The listing builds one solid part. Answer for the finished solid, in the listing's coordinates (mm). Face numbers are marked on the shaded views. A direction names the side the tool comes from. Give positions to 0.01 mm unless a question says otherwise; leave off trailing zeros. Write each loop counter-clockwise with the first axis right and the second up, starting at its lowest first coordinate (ties: lowest second). Pieces come first, ordered by that corner, then holes. Notation, with made-up numbers: (-15.5, -17.5) -> (-1.5, -17.5) arc R21 cw to (-1.5, 11.5) -> close; hole circle Ø9 at (34, -2.75). An arc over 180 degrees is marked (long way). Use CSV: the item, a comma, the result in double quotes. Start each with the question number.
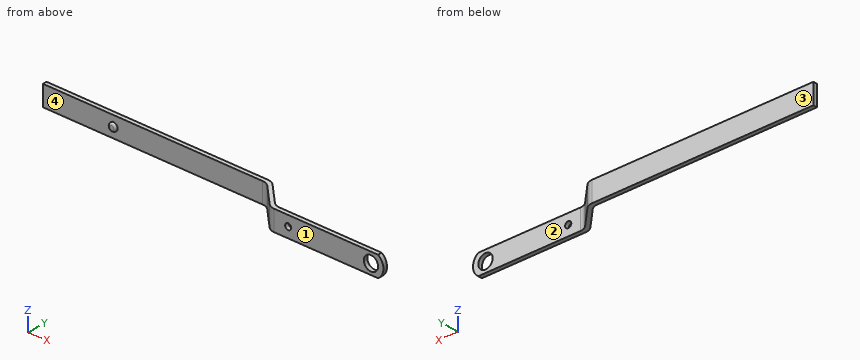
from build123d import *

# Parameters (mm, degrees)
SKETCH3_W           = 20
SKETCH3_H           = 4
FILLET1_R           = 10
BOSS_EXTRUDE1_DEPTH = 4
SKETCH4_4_R         = 7
SKETCH4_4_R_2       = 3
CUT_EXTRUDE6_DEPTH  = 4
SKETCH5_R           = 4
BOSS_EXTRUDE2_DEPTH = 2
FILLET4_R           = 2


with BuildPart() as part:
    # Sweep1: sweep along a path in Sketch2
    with BuildLine(Plane.XY) as sweep1_path:
        Line((105, 0), (0, 0))
        Line((0, 0), (-24.748737342, 24.748737342))
        Line((-24.748737342, 24.748737342), (-159.748737342, 24.748737342))
        Line((-159.748737342, 24.748737342), (-244.748737342, 24.748737342))
    # Sketch3 → Sweep1 (sweep)
    with BuildSketch(Plane(origin=(105, 0, 0), x_dir=(0, 0, -1), z_dir=(1, 0, 0))):
        Rectangle(SKETCH3_W, SKETCH3_H)
    sweep(path=sweep1_path.line, transition=Transition.RIGHT)

    # Fillet1
    fillet1_edges = [part.edges().sort_by_distance(p)[0] for p in [
        (-0.828427125, -2, 0),
        (0.828427125, 2, 0),
        (-23.920310217, 26.748737342, 0),
        (-25.577164466, 22.748737342, 0),
    ]]
    fillet(fillet1_edges, radius=FILLET1_R)

    # Sketch4 → Boss-Extrude1 (add)
    with BuildSketch(Plane(origin=(0, 2, 0), x_dir=(1, 0, 0), z_dir=(0, 1, 0))):
        with BuildLine():
            ThreePointArc((105, -10), (110.206555616, 0), (105, 10))
            Line((105, 10), (105, 0))
            Line((105, 0), (105, -10))
        make_face()
    extrude(amount=-BOSS_EXTRUDE1_DEPTH)

    # Sketch4<4> → Cut-Extrude6 (cut)
    with BuildSketch(Plane(origin=(0, 2, 0), x_dir=(1, 0, 0), z_dir=(0, 1, 0))):
        with Locations(Location((98, 0, 0), (0, 0, 270))):
            Circle(SKETCH4_4_R)
        with Locations(Location((17, 0, 0), (0, 0, 270))):
            Circle(SKETCH4_4_R_2)
    extrude(amount=-CUT_EXTRUDE6_DEPTH, mode=Mode.SUBTRACT)

    # Sketch5 → Boss-Extrude2 (add)
    with BuildSketch(Plane.XZ.offset(-22.748737342)):
        with Locations(Location((-175.748737342, 0, 0), (0, 0, 180))):
            Circle(SKETCH5_R)
    extrude(amount=BOSS_EXTRUDE2_DEPTH)

    # Fillet4
    fillet4_edges = [part.edges().sort_by_distance(p)[0] for p in [
        (-171.748737342, 20.748737342, 0),
    ]]
    fillet(fillet4_edges, radius=FILLET4_R - 0.0001)  # a hair under: the kernel refuses the full size


solid = part.part
Q1. Section A-A on x = 17 is taken. Give the vertices of the cut face in (y, z), then the cut area to 3 significant figures.
Q2. Section B-B on x = 98 is taken. Give the vertices of the cut face in (y, z).
Q3. Straight lines are drawn through the part: L1, parallel to X at y = 0.7, z = 0; L2, parallel to X at y = 0.25, z = 0; L3, parallel to Y at x = -132, z = -8. For each, find the intervals that lie inside material, in ascending order.
Q4. Section C-C on x = -183.5 is taken. Give the vertices of the cut face in (y, z), then the cut area to 3 significant figures.
Q5. Flat-ended cylindrical pins translate along their axes: pin 1 Ø1 at (y, z) = (7.5, -7.5) entering from -X; pin 2 Ø12 at (y, z) = (10, 4) entering from +X; pin 3 Ø3 at (y, z) = (15.5, 1) entering from +X. Find the tip coordinate at first contact, or state that the pin passes through.
Q6. Section D-D on y = 9.75 is taken. Give the vertices of the cut face in (x, z), then the cut area to 3 significant figures.
Q7. The mould has two halves that part along X. Classify the marked faces 3 and 4: +X half, -X half, draft (parallel to the pull), parting line (faces both ways), or undercut.
Q8. For the marked faces 1 and 2, determine the directions among +Z, -Z, +X, -X, +Y, -Y from which every point of the face is accessible in a straight line to the end or side of a thin tool.
Output:
1,outline,"(-2, -10) -> (2, -10) -> (2, -3) -> (-2, -3) -> close; (-2, 3) -> (2, 3) -> (2, 10) -> (-2, 10) -> close"
1,area,"56.0 mm²"
2,outline,"(-2, -10) -> (2, -10) -> (2, -7) -> (-2, -7) -> close; (-2, 7) -> (2, 7) -> (2, 10) -> (-2, 10) -> close"
3,L1,"-3.52 to 14, 20 to 91, 105 to 110.21"
3,L2,"-3.01 to 14, 20 to 91, 105 to 110.21"
3,L3,"22.75 to 26.75"
4,outline,"(22.75, -10) -> (26.75, -10) -> (26.75, 10) -> (22.75, 10) -> close"
4,area,"80.0 mm²"
5,pin 1,"x = -10.83"
5,pin 2,"x = -1.03"
5,pin 3,"x = -11.17"
6,outline,"(-12.58, -10) -> (-6.92, -10) -> (-6.92, 10) -> (-12.58, 10) -> close"
6,area,"113 mm²"
7,face 3,"draft"
7,face 4,"undercut"
8,face 1,"+Z, -Z, +X, -X, -Y"
8,face 2,"+Z, -Z, +X, +Y"
